For this review, take the finished solid that the model builds, in its own axes (mm). A direction names the side the tool comes from. Round coordinates to 2 decimals unless told otherwise and drop trailing zeros. Loops run counter-clockwise (first coordinate to the right, second up) from the corner with the lowest first, then second, coordinate; pieces in that order, holes last. Notation, with made-up numbers: M 27.25,1 L 36.25,1 A27 ccw 36.25,18 Z; hole C 53.25,50.5 d6. An arc over 180 degrees is marked long. Write item = value, one per line. Start each with the question number.
```python
from build123d import *

# Parameters (mm, degrees)
SKETCH1_W           = 80
SKETCH1_H           = 80
SKETCH1_R           = 2.5
BOSS_EXTRUDE1_DEPTH = 9.5
SKETCH3_R           = 5
CUT_EXTRUDE1_DEPTH  = 4.75
SKETCH10_R          = 7.25
SKETCH10_R_2        = 5
BOSS_EXTRUDE3_DEPTH = 10


with BuildPart() as part:
    # Sketch1 → Boss-Extrude1 (new body)
    with BuildSketch(Plane(origin=(0, 0, 0), x_dir=(1, 0, 0), z_dir=(0, 1, 0))):
        with Locations((40, 40)):
            Rectangle(SKETCH1_W, SKETCH1_H)
        with Locations((5, 75)):
            Circle(SKETCH1_R, mode=Mode.SUBTRACT)
        with Locations((75, 75)):
            Circle(SKETCH1_R, mode=Mode.SUBTRACT)
        with Locations((75, 5)):
            Circle(SKETCH1_R, mode=Mode.SUBTRACT)
        with Locations((5, 5)):
            Circle(SKETCH1_R, mode=Mode.SUBTRACT)
    extrude(amount=BOSS_EXTRUDE1_DEPTH)

    # Sketch3 → Cut-Extrude1 (cut, symmetric)
    with BuildSketch(Plane(origin=(0, 9.5, 0), x_dir=(1, 0, 0), z_dir=(0, 1, 0))):
        with Locations((40, 40)):
            Circle(SKETCH3_R)
    extrude(amount=CUT_EXTRUDE1_DEPTH, both=True, mode=Mode.SUBTRACT)

    # Sketch10 → Boss-Extrude3 (add)
    with BuildSketch(Plane(origin=(0, 4.75, 0), x_dir=(1, 0, 0), z_dir=(0, 1, 0))):
        with Locations((40, 40)):
            Circle(SKETCH10_R)
        with Locations((40, 40)):
            Circle(SKETCH10_R_2, mode=Mode.SUBTRACT)
    extrude(amount=BOSS_EXTRUDE3_DEPTH)


solid = part.part
```
(1) For pin 1 Ø5 at (x, z) = (41.5, -39.5) entering from +Y; pin 2 Ø24 at (x, z) = (27.5, -33.5) entering from +Y; pin 3 Ø12 at (x, z) = (66, -48) entering from +Y, all flat-tipped, find the tip position at first contact; note any pin that passes through.
(2) Add section D-D on z = -40. Write out the cut boundary in (x, y).
(3) Tool access review of faces 1 (the flat face through (39, 0, -41)), 2 (the cylindrical face through (34.247, 12.088, -35.588)): name each direction out of +Z, -Z, +X, -X, +Y, -Y from which nothing blocks a thin tool from reaching the whole face with its end or side.
(4) Add section C-C on x = 40. Write out the cut boundary in (y, z), and give its area (3 significant figures).
(5) Add section A-A on x = 5. Write out the cut boundary in (y, z).
(6) Draft analysis for pull direction X (two halves, no side actions). For faces 3 (the flat face through (39, 5, -80)), 4 (the cylindrical face through (36, 10, -43)), 5 (the flat face through (80, 5, -39)), state which applies: +X half, -X half, draft (parallel to the pull), parting line (faces both ways), or undercut.
(7) Wall thickness on L1, parallel to X at y = 3.5, z = -5; L2, parallel to Z at x = 75, y = 4; L3, parallel to X at y = 8.5, z = -40: over which ranges is each line inside the solid? List them lowest first.
(8) Add section B-B on z = -5. Write out the cut boundary in (x, y).
Answer sheet:
q1.pin_1 = 4.75
q1.pin_2 = 14.75
q1.pin_3 = 9.5
q2.outline = M 0,0 L 80,0 L 80,9.5 L 47.25,9.5 L 47.25,14.75 L 45,14.75 L 45,4.75 L 35,4.75 L 35,14.75 L 32.75,14.75 L 32.75,9.5 L 0,9.5 Z
q3.face_1 = +Z, -Z, +X, -X, -Y
q3.face_2 = +Y
q4.outline = M 0,-80 L 9.5,-80 L 9.5,-47.25 L 14.75,-47.25 L 14.75,-45 L 4.75,-45 L 4.75,-35 L 14.75,-35 L 14.75,-32.75 L 9.5,-32.75 L 9.5,0 L 0,0 Z
q4.area = 736 mm²
q5.outline = M 0,-80 L 9.5,-80 L 9.5,-77.5 L 0,-77.5 Z; M 0,-72.5 L 9.5,-72.5 L 9.5,-7.5 L 0,-7.5 Z; M 0,-2.5 L 9.5,-2.5 L 9.5,0 L 0,0 Z
q6.face_3 = draft
q6.face_4 = undercut
q6.face_5 = +X half
q7.L1 = 0 to 2.5, 7.5 to 72.5, 77.5 to 80
q7.L2 = -80 to -77.5, -72.5 to -7.5, -2.5 to 0
q7.L3 = 0 to 35, 45 to 80
q8.outline = M 0,0 L 2.5,0 L 2.5,9.5 L 0,9.5 Z; M 7.5,0 L 72.5,0 L 72.5,9.5 L 7.5,9.5 Z; M 77.5,0 L 80,0 L 80,9.5 L 77.5,9.5 Z
